Input: dimensioned drawing with shaded views. Units: mm. Origin: part minimum x, y, z. Give positions to 0.01 mm unless a question says otherwise; leave off trailing zeros. Write each loop counter-clockwise with the first axis right and the second up, starting at its lowest first coordinate (ties: lowest second). Pieces come first, ordered by that corner, then holes. Notation, with made-up numbers: M 56,54.5 L 99,54.5 A21 cw 99,79.5 Z; hole C -3.75,-18 d9. An arc over 180 degrees is marked long. Answer as a JSON object with one key per item and string values.
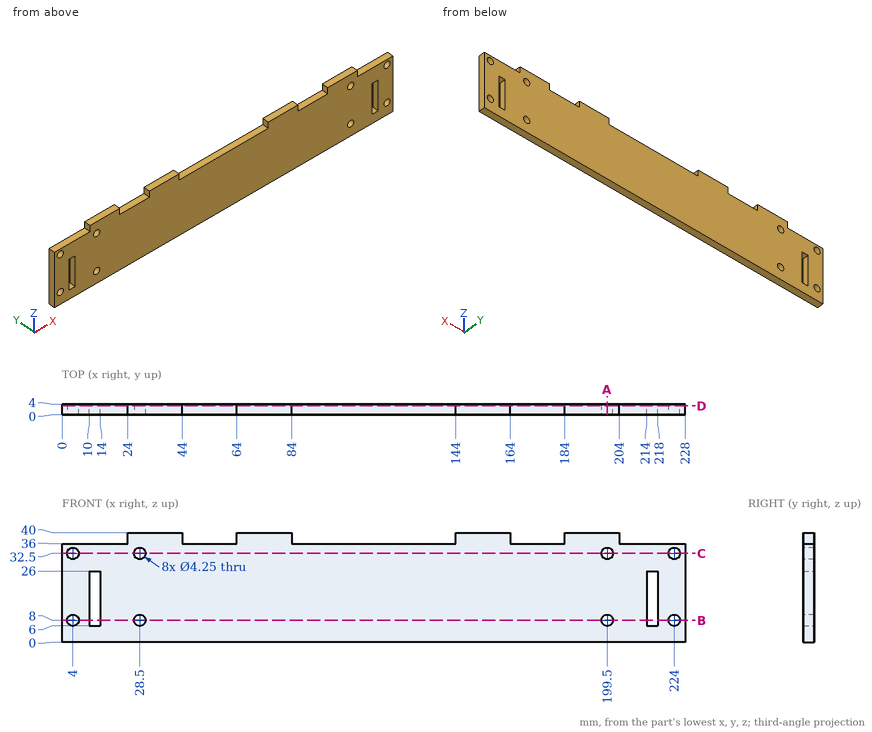
1) Cut plane A-A on x = 199.5. Return loops of the section in (y, z) (3 decimals).
Geometry check:
{"outline": "M 0,0 L 4,0 L 4,5.875 L 0,5.875 Z; M 0,10.125 L 4,10.125 L 4,30.375 L 0,30.375 Z; M 0,34.625 L 4,34.625 L 4,40 L 0,40 Z"}
2) Cut plane C-C on z = 32.5. Return loops of the section in (x, y) (3 decimals), and give its area (3 significant figures).
Geometry check:
{"outline": "M 0,0 L 1.875,0 L 1.875,4 L 0,4 Z; M 6.125,0 L 26.375,0 L 26.375,4 L 6.125,4 Z; M 30.625,0 L 197.375,0 L 197.375,4 L 30.625,4 Z; M 201.625,0 L 221.875,0 L 221.875,4 L 201.625,4 Z; M 226.125,0 L 228,0 L 228,4 L 226.125,4 Z", "area": "844 mm2"}
3) Line query: line 1 (X direction, y = 2.65, z = 32.5) (3 decimals); line 2 (Z direction, x = 224, y = 2) (3 decimals); line 3 (X direction, y = 2.6, z = 38). Output: solid intervals per line, ascending. Write a range as from..to.
Geometry check:
{"line 1": "x = 0..1.875, 6.125..26.375, 30.625..197.375, 201.625..221.875, 226.125..228", "line 2": "z = 0..5.875, 10.125..30.375, 34.625..36", "line 3": "x = 24..44, 64..84, 144..164, 184..204"}
4) Cut plane D-D on y = 3.35. Give the number of separate pieces and of enclosed holes in the cut face, and give its area (3 significant figures).
Geometry check:
{"separate pieces": "1", "enclosed holes": "10", "area": "8,250 mm2"}
5) Cut plane B-B on z = 8. Return loops of the section in (x, y) (3 decimals).
Geometry check:
{"outline": "M 0,0 L 1.875,0 L 1.875,4 L 0,4 Z; M 6.125,0 L 10,0 L 10,4 L 6.125,4 Z; M 14,0 L 26.375,0 L 26.375,4 L 14,4 Z; M 30.625,0 L 197.375,0 L 197.375,4 L 30.625,4 Z; M 201.625,0 L 214,0 L 214,4 L 201.625,4 Z; M 218,0 L 221.875,0 L 221.875,4 L 218,4 Z; M 226.125,0 L 228,0 L 228,4 L 226.125,4 Z"}
6) Contact query for flat-ended pins moving along their axis: P1, Ø1.2, axis at y = 3, z = 39, coming from the -X side; P2, Ø1.2, axis at y = 1.5, z = 38.5, coming from the +X side; P3, Ø1.2, axis at x = 49, y = 1.5, coming from the +Z side. Output: stop coordinate, or through.
Geometry check:
{"P1": "stops at x = 24", "P2": "stops at x = 204", "P3": "stops at z = 36"}
